from build123d import *

# Parameters (mm, degrees)
SKETCH1_R           = 6.35
SKETCH1_R_2         = 1.016
SKETCH1_R_3         = 0.080960071
SKETCH1_R_4         = 0.080960069
SKETCH1_R_5         = 0.080960077
BOSS_EXTRUDE1_DEPTH = 2.54
CUT_EXTRUDE1_DEPTH  = 2.54
CUT_EXTRUDE2_DEPTH  = 2.54


with BuildPart() as part:
    # Sketch1 → Boss-Extrude1 (new body)
    with BuildSketch(Plane(origin=(0, 0, 0), x_dir=(1, 0, 0), z_dir=(0, 1, 0))):
        with BuildLine():
            Line((-32.968194559, 49.876062167), (32.968194559, 49.876062167))
            ThreePointArc((32.968194559, 49.876062167), (34.552819694, 49.622589198), (35.979311114, 48.887464993))
            ThreePointArc((35.979311114, 48.887464993), (46.601053925, 38.895203237), (54.533013494, 26.657935048))
            ThreePointArc((54.533013494, 26.657935048), (56.406830639, 24.579655731), (59.096893531, 23.808943565))
            Line((59.096893531, 23.808943565), (71.51687593, 23.808943565))
            Line((71.51687593, 23.808943565), (76.59687593, 18.728943565))
            Line((76.59687593, 18.728943565), (76.59687593, -18.728943565))
            Line((76.59687593, -18.728943565), (71.51687593, -23.808943565))
            Line((71.51687593, -23.808943565), (59.096893531, -23.808943565))
            ThreePointArc((59.096893531, -23.808943565), (56.406830639, -24.579655731), (54.533013494, -26.657935048))
            ThreePointArc((54.533013494, -26.657935048), (45.317367474, -40.383551936), (32.740019521, -51.113463818))
            ThreePointArc((32.740019521, -51.113463818), (31.427532558, -51.711066727), (30, -51.915766654))
            Line((30, -51.915766654), (-30, -51.915766654))
            ThreePointArc((-30, -51.915766654), (-31.427532558, -51.711066727), (-32.740019521, -51.113463818))
            ThreePointArc((-32.740019521, -51.113463818), (-45.317367474, -40.383551936), (-54.533013494, -26.657935048))
            ThreePointArc((-54.533013494, -26.657935048), (-56.406830639, -24.579655731), (-59.096893531, -23.808943565))
            Line((-59.096893531, -23.808943565), (-71.51687407, -23.808943565))
            Line((-71.51687407, -23.808943565), (-76.59687407, -18.728943565))
            Line((-76.59687407, -18.728943565), (-76.59687407, 18.7325))
            Line((-76.59687407, 18.7325), (-71.51687407, 23.8125))
            Line((-71.51687407, 23.8125), (-59.09515487, 23.8125))
            ThreePointArc((-59.09515487, 23.8125), (-56.405221646, 24.583131223), (-54.531409104, 26.661216829))
            ThreePointArc((-54.531409104, 26.661216829), (-46.599883535, 38.896605459), (-35.979311114, 48.887464993))
            ThreePointArc((-35.979311114, 48.887464993), (-34.552819694, 49.622589198), (-32.968194559, 49.876062167))
        make_face()
        with Locations(Location((0, 0, 0), (0, 0, 270))):
            Circle(SKETCH1_R, mode=Mode.SUBTRACT)
        with Locations(Location((43.894926132, 35.273880181, 0), (0, 0, 270))):
            Circle(SKETCH1_R_2, mode=Mode.SUBTRACT)
        with Locations(Location((35.273880264, 43.894926065, 0), (0, 0, 90))):
            Circle(SKETCH1_R_2, mode=Mode.SUBTRACT)
        with Locations(Location((26.694927502, 26.694927451, 0), (0, 0, 270))):
            Circle(SKETCH1_R_3, mode=Mode.SUBTRACT)
        with Locations(Location((26.694927534, -26.694927601, 0), (0, 0, 270))):
            Circle(SKETCH1_R_3, mode=Mode.SUBTRACT)
        with Locations(Location((43.894926149, -35.273880364, 0), (0, 0, 90))):
            Circle(SKETCH1_R_2, mode=Mode.SUBTRACT)
        with Locations(Location((35.273880264, -43.894926232, 0), (0, 0, 270))):
            Circle(SKETCH1_R_2, mode=Mode.SUBTRACT)
        with Locations(Location((-26.694927518, -26.694927634, 0), (0, 0, 270))):
            Circle(SKETCH1_R_4, mode=Mode.SUBTRACT)
        with Locations(Location((-35.27388028, -43.894926248, 0), (0, 0, 90))):
            Circle(SKETCH1_R_2, mode=Mode.SUBTRACT)
        with Locations(Location((-43.894926149, -35.273880364, 0), (0, 0, 270))):
            Circle(SKETCH1_R_2, mode=Mode.SUBTRACT)
        with Locations(Location((-26.694927551, 26.694927419, 0), (0, 0, 270))):
            Circle(SKETCH1_R_5, mode=Mode.SUBTRACT)
        with Locations(Location((-43.894926165, 35.273880181, 0), (0, 0, 90))):
            Circle(SKETCH1_R_2, mode=Mode.SUBTRACT)
        with Locations(Location((-35.27388028, 43.894926049, 0), (0, 0, 270))):
            Circle(SKETCH1_R_2, mode=Mode.SUBTRACT)
    extrude(amount=BOSS_EXTRUDE1_DEPTH)

    # Sketch3 → Cut-Extrude1 (cut)
    with BuildSketch(Plane(origin=(0, 2.54, 0), x_dir=(1, 0, 0), z_dir=(0, 1, 0))):
        with BuildLine():
            Line((10.776307345, 12.572358569), (26.940768363, 28.736819587))
            ThreePointArc((26.940768363, 28.736819587), (28.736819587, 28.736819587), (28.736819587, 26.940768363))
            Line((28.736819587, 26.940768363), (12.572358569, 10.776307345))
            ThreePointArc((12.572358569, 10.776307345), (10.776307345, 10.776307345), (10.776307345, 12.572358569))
        make_face()
        with BuildLine():
            Line((16.51, -1.27), (39.37, -1.27))
            ThreePointArc((39.37, -1.27), (40.64, 0), (39.37, 1.27))
            Line((39.37, 1.27), (16.51, 1.27))
            ThreePointArc((16.51, 1.27), (15.24, 0), (16.51, -1.27))
        make_face()
        with BuildLine():
            Line((10.776307345, -12.572358569), (26.940768363, -28.736819587))
            ThreePointArc((26.940768363, -28.736819587), (28.736819587, -28.736819587), (28.736819587, -26.940768363))
            Line((28.736819587, -26.940768363), (12.572358569, -10.776307345))
            ThreePointArc((12.572358569, -10.776307345), (10.776307345, -10.776307345), (10.776307345, -12.572358569))
        make_face()
        with BuildLine():
            Line((-1.27, -16.51), (-1.27, -39.37))
            ThreePointArc((-1.27, -39.37), (0, -40.64), (1.27, -39.37))
            Line((1.27, -39.37), (1.27, -16.51))
            ThreePointArc((1.27, -16.51), (0, -15.24), (-1.27, -16.51))
        make_face()
        with BuildLine():
            Line((-12.572358569, -10.776307345), (-28.736819587, -26.940768363))
            ThreePointArc((-28.736819587, -26.940768363), (-28.736819587, -28.736819587), (-26.940768363, -28.736819587))
            Line((-26.940768363, -28.736819587), (-10.776307345, -12.572358569))
            ThreePointArc((-10.776307345, -12.572358569), (-10.776307345, -10.776307345), (-12.572358569, -10.776307345))
        make_face()
        with BuildLine():
            Line((-16.51, 1.27), (-39.37, 1.27))
            ThreePointArc((-39.37, 1.27), (-40.64, 0), (-39.37, -1.27))
            Line((-39.37, -1.27), (-16.51, -1.27))
            ThreePointArc((-16.51, -1.27), (-15.24, 0), (-16.51, 1.27))
        make_face()
        with BuildLine():
            Line((-10.776307345, 12.572358569), (-26.940768363, 28.736819587))
            ThreePointArc((-26.940768363, 28.736819587), (-28.736819587, 28.736819587), (-28.736819587, 26.940768363))
            Line((-28.736819587, 26.940768363), (-12.572358569, 10.776307345))
            ThreePointArc((-12.572358569, 10.776307345), (-10.776307345, 10.776307345), (-10.776307345, 12.572358569))
        make_face()
        with BuildLine():
            Line((1.27, 16.51), (1.27, 39.37))
            ThreePointArc((1.27, 39.37), (0, 40.64), (-1.27, 39.37))
            Line((-1.27, 39.37), (-1.27, 16.51))
            ThreePointArc((-1.27, 16.51), (0, 15.24), (1.27, 16.51))
        make_face()
    extrude(amount=-CUT_EXTRUDE1_DEPTH, mode=Mode.SUBTRACT)

    # Sketch4 → Cut-Extrude2 (cut)
    with BuildSketch(Plane(origin=(0, 2.54, 0), x_dir=(1, 0, 0), z_dir=(0, 1, 0))):
        with BuildLine():
            Line((44.59287593, 14.605), (67.45287593, 14.605))
            ThreePointArc((67.45287593, 14.605), (68.350901543, 14.233025612), (68.72287593, 13.335))
            Line((68.72287593, 13.335), (68.72287593, 12.065))
            ThreePointArc((68.72287593, 12.065), (68.350901543, 11.166974388), (67.45287593, 10.795))
            Line((67.45287593, 10.795), (44.59287593, 10.795))
            ThreePointArc((44.59287593, 10.795), (43.694850318, 11.166974388), (43.32287593, 12.065))
            Line((43.32287593, 12.065), (43.32287593, 13.335))
            ThreePointArc((43.32287593, 13.335), (43.694850318, 14.233025612), (44.59287593, 14.605))
        make_face()
        with BuildLine():
            Line((68.72287593, -13.335), (68.72287593, -12.065))
            ThreePointArc((68.72287593, -12.065), (68.350901543, -11.166974388), (67.45287593, -10.795))
            Line((67.45287593, -10.795), (44.59287593, -10.795))
            ThreePointArc((44.59287593, -10.795), (43.694850318, -11.166974388), (43.32287593, -12.065))
            Line((43.32287593, -12.065), (43.32287593, -13.335))
            ThreePointArc((43.32287593, -13.335), (43.694850318, -14.233025612), (44.59287593, -14.605))
            Line((44.59287593, -14.605), (67.45287593, -14.605))
            ThreePointArc((67.45287593, -14.605), (68.350901543, -14.233025612), (68.72287593, -13.335))
        make_face()
        with BuildLine():
            Line((-44.59287593, -14.605), (-67.45287593, -14.605))
            ThreePointArc((-67.45287593, -14.605), (-68.350901543, -14.233025612), (-68.72287593, -13.335))
            Line((-68.72287593, -13.335), (-68.72287593, -12.065))
            ThreePointArc((-68.72287593, -12.065), (-68.350901543, -11.166974388), (-67.45287593, -10.795))
            Line((-67.45287593, -10.795), (-44.59287593, -10.795))
            ThreePointArc((-44.59287593, -10.795), (-43.694850318, -11.166974388), (-43.32287593, -12.065))
            Line((-43.32287593, -12.065), (-43.32287593, -13.335))
            ThreePointArc((-43.32287593, -13.335), (-43.694850318, -14.233025612), (-44.59287593, -14.605))
        make_face()
        with BuildLine():
            Line((-68.72287593, 13.335), (-68.72287593, 12.065))
            ThreePointArc((-68.72287593, 12.065), (-68.350901543, 11.166974388), (-67.45287593, 10.795))
            Line((-67.45287593, 10.795), (-44.59287593, 10.795))
            ThreePointArc((-44.59287593, 10.795), (-43.694850318, 11.166974388), (-43.32287593, 12.065))
            Line((-43.32287593, 12.065), (-43.32287593, 13.335))
            ThreePointArc((-43.32287593, 13.335), (-43.694850318, 14.233025612), (-44.59287593, 14.605))
            Line((-44.59287593, 14.605), (-67.45287593, 14.605))
            ThreePointArc((-67.45287593, 14.605), (-68.350901543, 14.233025612), (-68.72287593, 13.335))
        make_face()
    extrude(amount=-CUT_EXTRUDE2_DEPTH, mode=Mode.SUBTRACT)


solid = part.part
Work out the finished part from the listing and answer in its coordinate system (mm). A direction names the side the tool comes from. Give positions to 0.01 mm unless a question says otherwise; leave off trailing zeros. Order: outer loops, then holes, each group sorted by start corner. A loop starts at its lowest first (then second) coordinate and runs counter-clockwise, first axis right, second up. Notation, with made-up numbers: M -8.5,68.25 L 0.5,68.25 A6 ccw 0.5,74.25 Z; hole C 46.5,-6 d5. An arc over 180 degrees is marked long. Return JSON: item names as keys, results as strings.
Q1. Each of these flat-tipped pins is pushed along its axis until it touches: pin 1 (1.3 mm diameter, centred on y = 1.5, z = -28.5, fed in from +X); pin 2 (0.8 mm diameter, centred on x = 60.5, y = 1, fed in from -Z). Where does it stop, or does it pass through?
Answer below:
{"pin 1": "stops at x = 53.93", "pin 2": "stops at z = -23.81"}
Q2. Find section B-B, the plane z = -22. Write down the section's boundary in (x, y), and give its area (3 significant figures).
Answer below:
{"outline": "M -73.33,0 L -23.8,0 L -23.8,2.54 L -73.33,2.54 Z; M -20.2,0 L -1.27,0 L -1.27,2.54 L -20.2,2.54 Z; M 1.27,0 L 20.2,0 L 20.2,2.54 L 1.27,2.54 Z; M 23.8,0 L 73.33,0 L 73.33,2.54 L 23.8,2.54 Z", "area": "348 mm^2"}
Q3. Which of the six approach directions +Z, -Z, +X, -X, +Y, -Y give full straight-line access (tool end or side, diameter ignored) to faces 4 (the face through (-74.021, 1.252, 21.305)), 5 (the face through (18.745, 1.288, 20.541))?
Answer below:
{"face 4": "+Z, -X, +Y, -Y", "face 5": "+Y, -Y"}
Q4. Find the intervals of material crossed by line 1 along Z through (x, y) = (60.5, 1) (3 decimals); line 2 along X through (y, z) = (0.5, 0); line 3 along Z through (x, y) = (27.5, 2.3), in increasing order. Write a range as [from, to].
Answer below:
{"line 1": "z = [-23.809, -14.605], [-10.795, 10.795], [14.605, 23.809]", "line 2": "x = [-76.6, -40.64], [-15.24, -6.35], [6.35, 15.24], [40.64, 76.6]", "line 3": "z = [-49.88, -29.06], [-25.7, -1.27], [1.27, 25.7], [29.06, 51.92]"}
Q5. Find section D-D, the plane y = 1.85. State how many separate pieces and enclosed holes the cut face has, and give its area (3 significant figures).
Answer below:
{"separate pieces": "1", "enclosed holes": "21", "area": "11,300 mm^2"}
Q6. Find section C-C, the plane x = -20. Write down the section's boundary in (y, z), and give its area (3 significant figures).
Answer below:
{"outline": "M 0,-49.88 L 2.54,-49.88 L 2.54,-21.8 L 0,-21.8 Z; M 0,-18.2 L 2.54,-18.2 L 2.54,-1.27 L 0,-1.27 Z; M 0,1.27 L 2.54,1.27 L 2.54,18.2 L 0,18.2 Z; M 0,21.8 L 2.54,21.8 L 2.54,51.92 L 0,51.92 Z", "area": "234 mm^2"}
Q7. The mould has two halves that part along X. Classify faces 1 (the face through (-20.541, 1.288, 18.745)), 2 (the face through (74.021, 1.252, -21.305)), 3 (the face through (-46.73, 1.25, -38.74)): pulls with the +X half, pulls with the -X half, needs draft (parallel to the pull), parting line crosses it, or undercut.
Answer below:
{"face 1": "undercut", "face 2": "pulls with the +X half", "face 3": "pulls with the -X half"}
Q8. Find section A-A, the plane x = -48. Write down the section's boundary in (y, z) (3 decimals).
Answer below:
{"outline": "M 0,-37.155 L 2.54,-37.155 L 2.54,-14.605 L 0,-14.605 Z; M 0,-10.795 L 2.54,-10.795 L 2.54,10.795 L 0,10.795 Z; M 0,14.605 L 2.54,14.605 L 2.54,37.155 L 0,37.155 Z"}
